```python
from build123d import *

# Parameters (mm, degrees)
CUT_EXTRUDE1_START                                  = -12.700000000000001
CUT_EXTRUDE1_DEPTH                                  = 12.700000000000001
BOSS_EXTRUDE1_DEPTH                                 = 12.700000000000001
CSK_FOR_5_16_FLAT_HEAD_MACHINE_SCREW_10_D           = 8.4328
CSK_FOR_5_16_FLAT_HEAD_MACHINE_SCREW_10_CSINK_D     = 16.129
CSK_FOR_5_16_FLAT_HEAD_MACHINE_SCREW_10_CSINK_ANGLE = 100


with BuildPart() as part:
    # Sketch1 → Revolve1 (revolve)
    with BuildSketch(Plane(origin=(0, 0, 0), x_dir=(1, 0, 0), z_dir=(0, 1, 0)), mode=Mode.PRIVATE) as revolve1_sk:
        Polygon((0, 0), (-116.39944919199999, -1.425e-14), (-116.39944919199999, -6.350000000000014), (-116.39944919199999, -22.86), (-109.82551422519657, -22.86), (-100.09689936468882, -22.86), (-100.09689936468882, -15.239999999999998), (-108.77944919199999, -15.239999999999998), (-108.77944919199999, -7.619999999999999), (0, -7.619999999999999), align=None)
    revolve(revolve1_sk.sketch.rotate(Axis((0, 0, 7.619999999999999), (0, 0, -1)), 180), axis=Axis((0, 0, 7.619999999999999), (0, 0, -1)))

    # Sketch2 → Cut-Extrude1 (cut)
    with BuildSketch(Plane.XY.offset(22.86).offset(CUT_EXTRUDE1_START)):
        with BuildLine():
            Line((-108.77944919199999, -1.239e-14), (-14.769960459073417, 0))
            Line((-14.769960459073417, 0), (-4.49e-15, 14.76996045907346))
            Line((-4.49e-15, 14.76996045907346), (9.3e-16, 108.77944919199999))
            ThreePointArc((9.3e-16, 108.77944919199999), (-76.91868617740069, 76.9186861774007), (-108.77944919199999, -1.239e-14))
        make_face()
        with BuildLine():
            Line((2.664e-14, -108.77944919199999), (0, -24.8599350617269))
            Line((0, -24.8599350617269), (26.65786083148447, 0))
            Line((26.65786083148447, 0), (108.77944919199999, -9.3e-16))
            ThreePointArc((108.77944919199999, -9.3e-16), (76.9186861774007, -76.91868617740069), (2.664e-14, -108.77944919199999))
        make_face()
    extrude(amount=CUT_EXTRUDE1_DEPTH, mode=Mode.SUBTRACT)

    # Sketch4 → Boss-Extrude1 (add)
    with BuildSketch(Plane.XY.offset(7.619999999999999)):
        with BuildLine():
            Line((0, 108.77944919199999), (4.3e-16, 100.09689936468882))
            ThreePointArc((4.3e-16, 100.09689936468882), (4.507744656252515, 99.99534739445967), (9.006342768425501, 99.69089754015798))
            Line((9.006342768425501, 99.69089754015798), (9.006342768425501, 108.40597011443852))
            ThreePointArc((9.006342768425501, 108.40597011443852), (4.507041620723805, 108.68603931666647), (0, 108.77944919199999))
        make_face()
        with BuildLine():
            Line((2.389e-14, -100.09689936468882), (2.664e-14, -108.77944919199999))
            ThreePointArc((2.664e-14, -108.77944919199999), (-4.5070416207237916, -108.68603931666647), (-9.006342768425498, -108.40597011443852))
            Line((-9.006342768425498, -108.40597011443852), (-9.006342768425498, -99.69089754015796))
            ThreePointArc((-9.006342768425498, -99.69089754015796), (-4.507744656252502, -99.99534739445966), (2.389e-14, -100.09689936468882))
        make_face()
    extrude(amount=BOSS_EXTRUDE1_DEPTH)

    # CSK for 5/16 Flat Head Machine Screw (100)1 (through all)
    with Locations(Plane(origin=(-71.265307908, 56.784373632, 7.62), x_dir=(1, 0, 0), z_dir=(0, 0, 1))):
        with Locations((0, 0), (142.072512407, -114.138963606)):
            CounterSinkHole(CSK_FOR_5_16_FLAT_HEAD_MACHINE_SCREW_10_D / 2, CSK_FOR_5_16_FLAT_HEAD_MACHINE_SCREW_10_CSINK_D / 2, counter_sink_angle=CSK_FOR_5_16_FLAT_HEAD_MACHINE_SCREW_10_CSINK_ANGLE)


solid = part.part
```
Build history of the part. All positions in model axes, mm. A direction names the side the tool comes from. Give positions to 0.01 mm unless a question says otherwise; leave off trailing zeros. Loops run counter-clockwise (first coordinate to the right, second up) from the corner with the lowest first, then second, coordinate; pieces in that order, holes last.
1) Drop flat-ended pins along their axis: P1, Ø3, axis at y = 86.5, z = 11.5, coming from the -X side; P2, Ø1.5, axis at x = 19.5, z = 19.5, coming from the +Y side; P3, Ø12, axis at x = -38.5, z = 8.5, coming from the +Y side. Give the stop position or say it passes through.
Values follow:
P1: stops at x = -79.52
P2: stops at y = 114.88
P3: stops at y = 111.77
2) Probe line 1 along X through (y, z) = (68, 11.5); line 2 along X through (y, z) = (93, 11); line 3 along Z through (x, y) = (2, 34). List the from-to ranges inside material, lowest first.
Values follow:
line 1: x = -94.47 to -84.91, 84.91 to 94.47
line 2: x = -70 to -56.43, 56.43 to 70
line 3: z = 0 to 7.62
3) 3-axis set-ups, long thin cutter, end or side, ignore diameter. For faces 1 (the face through (-104, 0, 19)), 2 (the face through (101.81, -38.31, 13.44)), 3 (the face through (111.024, -34.963, 11.59)): which of +Z, -Z, +X, -X, +Y, -Y reach the whole face in a straight line?
Values follow:
face 1: +Z
face 2: none
face 3: +Z, -Z
4) Band-saw the part on C-C on x = -95. List the corners of the cut face in (y, z), then the cut area to 3 significant figures.
Values follow:
outline: (-67.26, 0) - (67.26, 0) - (67.26, 22.86) - (52.99, 22.86) - (52.99, 7.62) - (-52.99, 7.62) - (-52.99, 15.24) - (-31.53, 15.24) - (-31.53, 22.86) - (-67.26, 22.86) - close
area: 1,620 mm2
5) Band-saw the part on A-A on z = 18.75. List the corners of the cut face in (x, y).
Values follow:
outline: circle Ø232.8 at (0, 0); hole (-108.78, 0) - (-100.1, 0) arc R100.1 ccw to (0, -100.1) - (0, -108.78) arc R108.78 ccw to (108.78, 0) - (100.1, 0) arc R100.1 ccw to (0, 100.1) - (0, 108.78) arc R108.78 ccw to start
6) Two-plate mould, pull along Z, no slides. Class faces 4 (the face through (-87, -52, 22.86)), 5 (the face through (2, -2, 0)), 6 (the face through (0, -104, 15)), 7 (the face through (-9.006, -104, 11)): released by +Z, released by -Z, zero draft, split by the parting line, or undercut.
Values follow:
face 4: released by +Z
face 5: released by -Z
face 6: zero draft
face 7: undercut
7) Band-saw the part on B-B on y = -17.5. List the corners of the cut face in (x, z), then the cut area to 3 significant figures.
Values follow:
outline: (-115.08, 0) - (115.08, 0) - (115.08, 22.86) - (107.36, 22.86) - (107.36, 7.62) - (-107.36, 7.62) - (-107.36, 15.24) - (-98.56, 15.24) - (-98.56, 22.86) - (-115.08, 22.86) - close
area: 2,060 mm2
